Input: part model. Units: mm. Frame: model coordinates. Coordinates: 2 decimals unless noted, no trailing zeros. Loops run counter-clockwise (first coordinate to the right, second up) from the corner with the lowest first, then second, coordinate; pieces in that order, holes last.
```python
from build123d import *

# Parameters (mm, degrees)
SKETCH_1_R          = 16
EXTRUDE_1_DEPTH     = 10
SKETCH_2_R          = 1.8
CUT_EXTRUDE_1_DEPTH = 20
FILLET_1_R          = 1
FILLET_2_R          = 0.5


with BuildPart() as part:
    # Эскиз1 → Бобышка-Вытянуть1 (new body)
    with BuildSketch(Plane(origin=(0, 0, 0), x_dir=(1, 0, 0), z_dir=(0, 1, 0))):
        with Locations(Location((0, 0, 0), (0, 0, 270))):
            Circle(SKETCH_1_R)
    extrude(amount=EXTRUDE_1_DEPTH)

    # Эскиз2 → Вырез-Вытянуть1 (cut)
    with BuildSketch(Plane(origin=(0, 10, 0), x_dir=(1, 0, 0), z_dir=(0, 1, 0))):
        with Locations(Location((0, 13.5, 0), (0, 0, 270))):
            Circle(SKETCH_2_R)
        with Locations(Location((11.691342951, -6.75, 0), (0, 0, 270))):
            Circle(SKETCH_2_R)
        with Locations(Location((-11.691342951, -6.75, 0), (0, 0, 270))):
            Circle(SKETCH_2_R)
    extrude(amount=-CUT_EXTRUDE_1_DEPTH, mode=Mode.SUBTRACT)

    # Скругление1
    # the kernel refuses this fillet: 1 mm, written as the material it takes off along each edge
    with BuildSketch(Plane(origin=(0, 10, 0), x_dir=(0, 0, 1), z_dir=(-1, 0, 0))) as fillet_1_piece_1:
        with BuildLine():
            CenterArc((16 - FILLET_1_R, -FILLET_1_R), FILLET_1_R, 0, 90)
            Line((16 - FILLET_1_R, 0), (16, 0))
            Line((16, 0), (16, -FILLET_1_R))
        make_face()
    revolve(axis=Axis((0, 10, 0), (0, 1, 0)), mode=Mode.SUBTRACT)

    # Скругление2
    fillet_2_edges = [part.edges().sort_by_distance(p)[0] for p in [
        (11.691342951, 0, 4.95),
        (-11.691342951, 0, 4.95),
        (0, 0, -15.3),
    ]]
    fillet(fillet_2_edges, radius=FILLET_2_R)


solid = part.part
```
Item 1: Mould query, pull axis X, two halves, no side actions, for faces 1 (the face through (0, 0, 0)), 2 (the face through (-0.689, 5.316, -11.837)), 3 (the face through (-15.62, 4.44, -3.47)). Classes: +X half, -X half, draft (parallel to the pull), parting line (faces both ways), or undercut.
Result:
face 1: draft
face 2: undercut
face 3: parting line
Item 2: Section query B-B (y = 2.25). Output: boundary loops of the cut face in (x, z).
Result:
outline: circle Ø32 at (0, 0); hole circle Ø3.6 at (-11.69, 6.75); hole circle Ø3.6 at (0, -13.5); hole circle Ø3.6 at (11.69, 6.75)
Item 3: Contact query for flat-ended pins moving along their axis: P1, Ø1.5, axis at y = 8, z = -9, coming from the +X side; P2, Ø1, axis at y = 2.5, z = -5, coming from the -X side; P3, Ø2, axis at x = 3, y = 6, coming from the +Z side; P4, Ø3, axis at x = 0, z = -13.5, coming from the -Y side. Output: stop coordinate, or through.
Result:
P1: stops at x = 13.71
P2: stops at x = -15.35
P3: stops at z = 15.87
P4: passes through
Item 4: Section query A-A (x = 0). Output: boundary loops of the cut face in (y, z), then the cut area to 3 significant figures.
Result:
outline: (0, -16) - (9, -16) arc R1 ccw to (9.95, -15.3) - (0.5, -15.3) arc R0.5 ccw to (0, -15.8) - close; (0, -11.2) arc R0.5 ccw to (0.5, -11.7) - (10, -11.7) - (10, 15) arc R1 ccw to (9, 16) - (0, 16) - close
area: 283 mm2
Item 5: Line query: L1, parallel to X at y = 6, z = 7; L2, parallel to X at y = 3, z = 6.75; L3, parallel to Y at x = -14, z = 6.5. Output: solid intervals per line, ascending.
Result:
L1: x = -14.39 to -13.47, -9.91 to 9.91, 13.47 to 14.39
L2: x = -14.51 to -13.49, -9.89 to 9.89, 13.49 to 14.51
L3: y = 0 to 9.9
